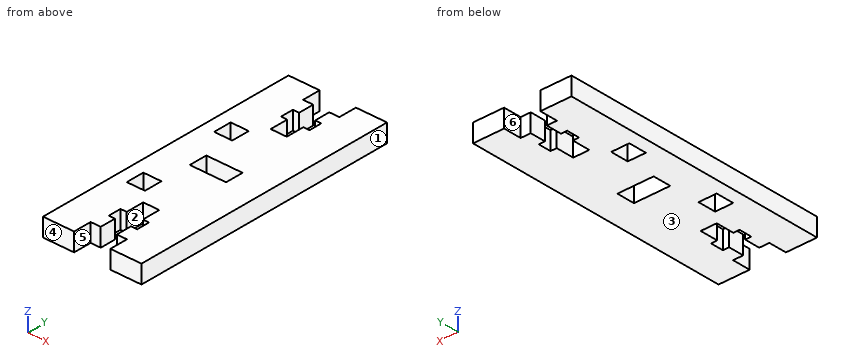
```python
from build123d import *

# Parameters (mm, degrees)
BOSS_EXTRUDE1_DEPTH = 3.5
SKETCH2_W           = 3.5
SKETCH2_H           = 3.5
CUT_EXTRUDE1_DEPTH  = 28.901612857
SKETCH3_W           = 7
SKETCH3_H           = 3.5
CUT_EXTRUDE2_DEPTH  = 28.901612857


with BuildPart() as part:
    # Sketch1 → Boss-Extrude1 (new body)
    with BuildSketch(Plane.XY):
        Polygon((3.5, 26), (3.5, 22.5), (1.55, 22.5), (1.55, 19.5), (2.75, 19.5), (2.75, 17), (1.55, 17), (1.55, 13.5), (-1.55, 13.5), (-1.55, 17), (-2.75, 17), (-2.75, 19.5), (-1.55, 19.5), (-1.55, 22.5), (-3.5, 22.5), (-3.5, 26), (-9.5, 26), (-9.5, -26), (-3.5, -26), (-3.5, -22.5), (-1.55, -22.5), (-1.55, -19.5), (-2.75, -19.5), (-2.75, -17), (-1.55, -17), (-1.55, -13.5), (1.55, -13.5), (1.55, -17), (2.75, -17), (2.75, -19.5), (1.55, -19.5), (1.55, -22.5), (3.5, -22.5), (3.5, -26), (9.5, -26), (9.5, 26), align=None)
    extrude(amount=BOSS_EXTRUDE1_DEPTH)

    # Sketch2 → Cut-Extrude1 (cut, through all)
    with BuildSketch(Plane(origin=(0, 0, 0), x_dir=(-1, 0, 0), z_dir=(0, 0, -1))):
        with Locations((5.25, -9.25)):
            Rectangle(SKETCH2_W, SKETCH2_H)
        with Locations((5.25, 9.25)):
            Rectangle(SKETCH2_W, SKETCH2_H)
    extrude(amount=-CUT_EXTRUDE1_DEPTH, mode=Mode.SUBTRACT)

    # Sketch3 → Cut-Extrude2 (cut, through all)
    with BuildSketch(Plane(origin=(0, 0, 0), x_dir=(-1, 0, 0), z_dir=(0, 0, -1))):
        with Locations((0, 0.25)):
            Rectangle(SKETCH3_W, SKETCH3_H)
    extrude(amount=-CUT_EXTRUDE2_DEPTH, mode=Mode.SUBTRACT)


solid = part.part
```
The listing builds one solid part. Answer for the finished solid, in the listing's coordinates (mm). Face numbers are marked on the shaded views. A direction names the side the tool comes from. Give positions to 0.01 mm unless a question says otherwise; leave off trailing zeros. Write each loop counter-clockwise with the first axis right and the second up, starting at its lowest first coordinate (ties: lowest second). Pieces come first, ordered by that corner, then holes. Notation, with made-up numbers: M -20,62.25 L 28,62.25 A26 cw 28,82.25 Z; hole C 14,65 d6. An arc over 180 degrees is marked long. Write each question's results on one line, items separated by ' | '.
Q1. A tool of negligible diameter and unlimited length cuts with its end or side. For the marked faces 4, 5 and 6, from which of +Z, -Z, +X, -X, +Y, -Y can it reach the whole face along a straight path? Write none if from no direction.
Output values:
face 4: +Z, -Z, +X, -X, -Y | face 5: +Z, -Z, -Y | face 6: +Z, -Z, +Y
Q2. For a pull along X with two mould halves and no side action, classify the marked faces 1, 2 and 3 as released by +X, released by -X, zero draft, split by the parting line, or undercut.
Output values:
face 1: released by +X | face 2: undercut | face 3: zero draft
Q3. Section C-C, the plane x = -4 is taken. Write down the section's boundary in (y, z), then the cut area to 4 significant figures.
Output values:
outline: M -26,0 L -11,0 L -11,3.5 L -26,3.5 Z; M -7.5,0 L 7.5,0 L 7.5,3.5 L -7.5,3.5 Z; M 11,0 L 26,0 L 26,3.5 L 11,3.5 Z | area: 157.5 mm2
Q4. Flat-ended cylindrical pins translate along their axes: P1, Ø5, axis at x = -1, y = 14, coming from the -Z side; P2, Ø1.3, axis at x = 2.5, z = 2, coming from the +Y side; P3, Ø1.6, axis at x = 0.5, z = 2, coming from the +Y side. Find the tip coordinate at first contact, or state that the pin passes through.
Output values:
P1: z = 0 | P2: y = 22.5 | P3: y = 13.5
Q5. Section B-B, the plane x = 2.25 is taken. Write down the section's boundary in (y, z).
Output values:
outline: M -22.5,0 L -19.5,0 L -19.5,3.5 L -22.5,3.5 Z; M -17,0 L -1.5,0 L -1.5,3.5 L -17,3.5 Z; M 2,0 L 17,0 L 17,3.5 L 2,3.5 Z; M 19.5,0 L 22.5,0 L 22.5,3.5 L 19.5,3.5 Z
Q6. Consider L1, parallel to Y at x = 2, z = 0.7; L2, parallel to Y at x = -4.75, z = 1.55; L3, parallel to Y at x = 3.25, z = 2.8. Determine where each line is inside the solid, lowest interval first. Write a range as from..to.
Output values:
L1: -22.5..-19.5, -17..-1.5, 2..17, 19.5..22.5 | L2: -26..-11, -7.5..7.5, 11..26 | L3: -22.5..-1.5, 2..22.5
Q7. Section D-D, the plane y = -18 is taken. Write down the section's boundary in (x, z).
Output values:
outline: M -9.5,0 L -2.75,0 L -2.75,3.5 L -9.5,3.5 Z; M 2.75,0 L 9.5,0 L 9.5,3.5 L 2.75,3.5 Z
Q8. Section A-A, the plane y = -9 is taken. Write down the section's boundary in (x, z), then the cut area to 4 significant figures.
Output values:
outline: M -9.5,0 L -7,0 L -7,3.5 L -9.5,3.5 Z; M -3.5,0 L 9.5,0 L 9.5,3.5 L -3.5,3.5 Z | area: 54.25 mm2
